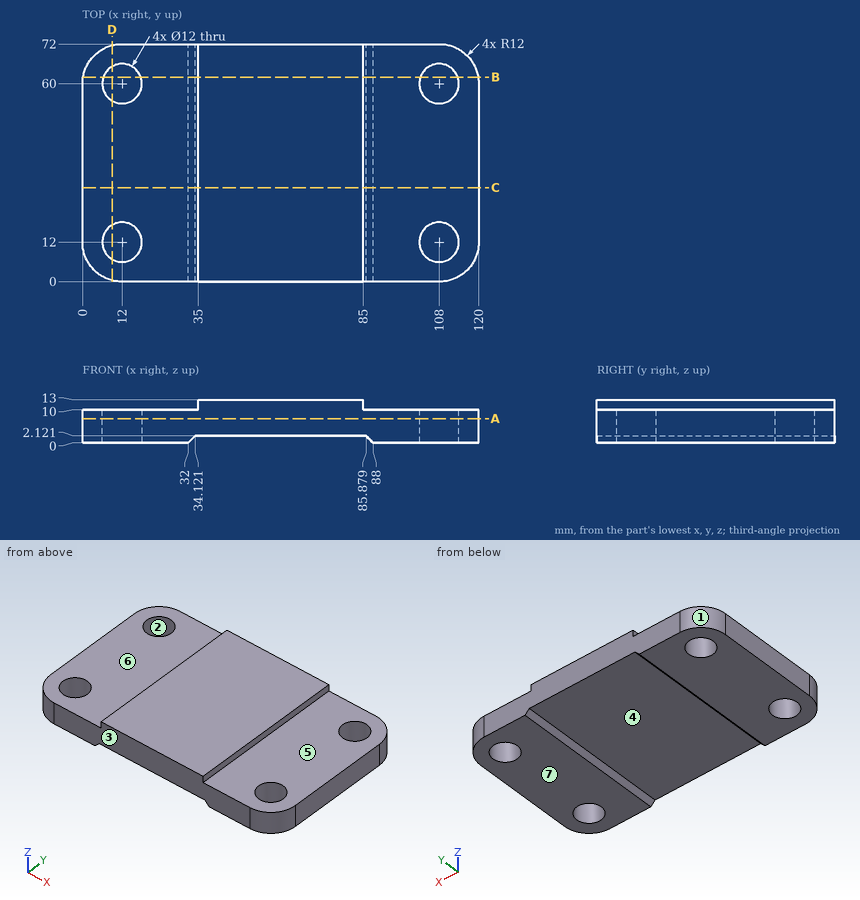
Part print with two shaded views. Sizes in mm from the minimum x, y, z corner. A direction names the side the tool comes from. Round coordinates to 2 decimals unless told otherwise and drop trailing zeros. Order: outer loops, then holes, each group sorted by start corner. A loop starts at its lowest first (then second) coordinate and runs counter-clockwise, first axis right, second up. Notation, with made-up numbers: (-3, 86.5) - (23, 86.5) arc R28 cw to (23, 108.5) - close; hole circle Ø7 at (50, 56.5). An arc over 180 degrees is marked (long way). Return JSON: item names as keys, results as strings.
(1) Cut at D-D (x = 9). Give the cut face in (y, z).
Answer key:
{"outline": "(0.38, 0) - (6.8, 0) - (6.8, 10) - (0.38, 10) - close; (17.2, 0) - (54.8, 0) - (54.8, 10) - (17.2, 10) - close; (65.2, 0) - (71.62, 0) - (71.62, 10) - (65.2, 10) - close"}
(2) Pin check, flat tips, straight feed: pin 1 Ø5 at (x, y) = (29.5, 57) entering from -Z; pin 2 Ø2 at (x, y) = (23, 57.5) entering from +Z; pin 3 Ø1 at (x, y) = (57, 44.5) entering from -Z; pin 4 Ø4 at (y, z) = (64, 9) entering from +X. Stop position of each tip, or through.
Answer key:
{"pin 1": "stops at z = 0", "pin 2": "stops at z = 10", "pin 3": "stops at z = 2.12", "pin 4": "stops at x = 119.83"}
(3) Wall check: probe 1 along Y at (x, z) = (108, 7.75); probe 2 along Y at (x, z) = (113, 9) (1 decimal); probe 3 along X at (y, z) = (63, 4.25) (1 decimal). Give the ranges that are in metal, low to high. Write a range as from..to.
Answer key:
{"probe 1": "y = 0..6, 18..54, 66..72", "probe 2": "y = 1.1..8.7, 15.3..56.7, 63.3..70.9", "probe 3": "x = 0.4..6.8, 17.2..102.8, 113.2..119.6"}
(4) Cut at A-A (z = 7.25). Give the cut face in (x, y).
Answer key:
{"outline": "(0, 12) arc R12 ccw to (12, 0) - (108, 0) arc R12 ccw to (120, 12) - (120, 60) arc R12 ccw to (108, 72) - (12, 72) arc R12 ccw to (0, 60) - close; hole circle Ø12 at (12, 12); hole circle Ø12 at (12, 60); hole circle Ø12 at (108, 12); hole circle Ø12 at (108, 60)"}
(5) Cut at C-C (y = 28.5). Give the cut face in (x, z).
Answer key:
{"outline": "(0, 0) - (32, 0) - (34.12, 2.12) - (85.88, 2.12) - (88, 0) - (120, 0) - (120, 10) - (85, 10) - (85, 13) - (35, 13) - (35, 10) - (0, 10) - close"}
(6) Tool access for the marked faces 4, 5, 6 and 7: list every direction of +Z, -Z, +X, -X, +Y, -Y with a clear straight run to the whole face (end or side of a thin tool).
Answer key:
{"face 4": "-Z, +Y, -Y", "face 5": "+Z, +X, +Y, -Y", "face 6": "+Z, -X, +Y, -Y", "face 7": "-Z, +X, -X, +Y, -Y"}
(7) Cut at B-B (y = 62). Give the cut face in (x, z).
Answer key:
{"outline": "(0.17, 0) - (6.34, 0) - (6.34, 10) - (0.17, 10) - close; (17.66, 0) - (32, 0) - (34.12, 2.12) - (85.88, 2.12) - (88, 0) - (102.34, 0) - (102.34, 10) - (85, 10) - (85, 13) - (35, 13) - (35, 10) - (17.66, 10) - close; (113.66, 0) - (119.83, 0) - (119.83, 10) - (113.66, 10) - close"}
(8) Pull direction X, two halves, no side cores. Call the marked faces 1, 2 and 3: +X half, -X half, draft (parallel to the pull), parting line (faces both ways), or undercut.
Answer key:
{"face 1": "-X half", "face 2": "undercut", "face 3": "draft"}
